from build123d import *

# Parameters (mm, degrees)
EXTRUDE_1_DEPTH          = 85
SKETCH_2_W               = 59.36627173602581
SKETCH_2_H               = 8.418969471425655
EXTRUDE_2_DEPTH          = 25
FILLET_1_R               = 6
FILLET_2_R               = 5
CUT_EXTRUDE_1_REACH      = 117.911
SKETCH_4_R               = 1.499999999999997
SKETCH_7_W               = 35.37461908353682
SKETCH_7_H               = 31.585915090625495
CUT_EXTRUDE_2_DEPTH      = 123.13645897424483
FILLET_3_R               = 5
FILLET_4_R               = 0.5
CUT_EXTRUDE_3_DEPTH      = 192.29117767705227
CUT_EXTRUDE_3_DEPTH_BACK = 192.29117767705227
SKETCH_9_R               = 1.8999999999999981
CUT_EXTRUDE_4_DEPTH      = 27.999999999999996


with BuildPart() as part:
    # 草图1 → 凸台-拉伸1 (new, symmetric)
    with BuildSketch(Plane.XY):
        Polygon((-37.5, 10.529999999999998), (-3.5592322501332707, 10.529999999999998), (-8.298471778986107, 19.8329163418583), (-23.723742156818243, 50.11203580857437), (-19.449282757937613, 61.53100528), (-37.5, 61.53100528), align=None)
    extrude(amount=EXTRUDE_1_DEPTH, both=True)

    # 草图2 → 凸台-拉伸2 (add)
    with BuildSketch(Plane.ZY.offset(37.5)):
        with Locations((0, 54.32152054428719)):
            Rectangle(SKETCH_2_W, SKETCH_2_H)
    extrude(amount=EXTRUDE_2_DEPTH)

    # 圆角1
    fillet_1_edges = [part.edges().sort_by_distance(p)[0] for p in [
        (-37.5, 54.32152054428719, -29.683135868012904),
        (-37.5, 54.32152054428719, 29.683135868012904),
    ]]
    fillet(fillet_1_edges, radius=FILLET_1_R)

    # 圆角2
    fillet_2_edges = [part.edges().sort_by_distance(p)[0] for p in [
        (-62.5, 54.32152054428719, -29.683135868012904),
        (-62.5, 54.32152054428719, 29.683135868012904),
    ]]
    fillet(fillet_2_edges, radius=FILLET_2_R)

    # 草图4 → 切除-拉伸1 (cut, up to next)
    with BuildSketch(Plane(origin=(0, 58.53100528000001, 0), x_dir=(1, 0, 0), z_dir=(0, 1, 0)), mode=Mode.PRIVATE) as cut_extrude_1_sk1:
        with Locations(Location((-47.387450092880144, 14.526154223892442, 0), (0, 0, 270))):
            Circle(SKETCH_4_R)
    cut_extrude_1_tool1 = extrude(cut_extrude_1_sk1.sketch, amount=-CUT_EXTRUDE_1_REACH, mode=Mode.PRIVATE) & part.part
    # 草图4 → 切除-拉伸1 (cut, up to next)
    with BuildSketch(Plane(origin=(0, 58.53100528000001, 0), x_dir=(1, 0, 0), z_dir=(0, 1, 0)), mode=Mode.PRIVATE) as cut_extrude_1_sk2:
        with Locations(Location((-52.407927387117596, 7.976309366063233, 0), (0, 0, 270))):
            Circle(SKETCH_4_R)
    cut_extrude_1_tool2 = extrude(cut_extrude_1_sk2.sketch, amount=-CUT_EXTRUDE_1_REACH, mode=Mode.PRIVATE) & part.part
    # 草图4 → 切除-拉伸1 (cut, up to next)
    with BuildSketch(Plane(origin=(0, 58.53100528000001, 0), x_dir=(1, 0, 0), z_dir=(0, 1, 0)), mode=Mode.PRIVATE) as cut_extrude_1_sk3:
        with Locations(Location((-59.01827910600927, -2.429e-14, 0), (0, 0, 270))):
            Circle(SKETCH_4_R)
    cut_extrude_1_tool3 = extrude(cut_extrude_1_sk3.sketch, amount=-CUT_EXTRUDE_1_REACH, mode=Mode.PRIVATE) & part.part
    # 草图4 → 切除-拉伸1 (cut, up to next)
    with BuildSketch(Plane(origin=(0, 58.53100528000001, 0), x_dir=(1, 0, 0), z_dir=(0, 1, 0)), mode=Mode.PRIVATE) as cut_extrude_1_sk4:
        with Locations(Location((-47.387450092880144, -2.456e-14, 0), (0, 0, 270))):
            Circle(SKETCH_4_R)
    cut_extrude_1_tool4 = extrude(cut_extrude_1_sk4.sketch, amount=-CUT_EXTRUDE_1_REACH, mode=Mode.PRIVATE) & part.part
    # 草图4 → 切除-拉伸1 (cut, up to next)
    with BuildSketch(Plane(origin=(0, 58.53100528000001, 0), x_dir=(1, 0, 0), z_dir=(0, 1, 0)), mode=Mode.PRIVATE) as cut_extrude_1_sk5:
        with Locations(Location((-52.407927387117596, -7.976309366063282, 0), (0, 0, 270))):
            Circle(SKETCH_4_R)
    cut_extrude_1_tool5 = extrude(cut_extrude_1_sk5.sketch, amount=-CUT_EXTRUDE_1_REACH, mode=Mode.PRIVATE) & part.part
    # 草图4 → 切除-拉伸1 (cut, up to next)
    with BuildSketch(Plane(origin=(0, 58.53100528000001, 0), x_dir=(1, 0, 0), z_dir=(0, 1, 0)), mode=Mode.PRIVATE) as cut_extrude_1_sk6:
        with Locations(Location((-47.387450092880144, -14.52615422389249, 0), (0, 0, 270))):
            Circle(SKETCH_4_R)
    cut_extrude_1_tool6 = extrude(cut_extrude_1_sk6.sketch, amount=-CUT_EXTRUDE_1_REACH, mode=Mode.PRIVATE) & part.part
    add(cut_extrude_1_tool1.solids().sort_by_distance((-47.38745, 58.531005, -14.526154))[0], mode=Mode.SUBTRACT)
    add(cut_extrude_1_tool2.solids().sort_by_distance((-52.407927, 58.531005, -7.976309))[0], mode=Mode.SUBTRACT)
    add(cut_extrude_1_tool3.solids().sort_by_distance((-59.018279, 58.531005, 0))[0], mode=Mode.SUBTRACT)
    add(cut_extrude_1_tool4.solids().sort_by_distance((-47.38745, 58.531005, 0))[0], mode=Mode.SUBTRACT)
    add(cut_extrude_1_tool5.solids().sort_by_distance((-52.407927, 58.531005, 7.976309))[0], mode=Mode.SUBTRACT)
    add(cut_extrude_1_tool6.solids().sort_by_distance((-47.38745, 58.531005, 14.526154))[0], mode=Mode.SUBTRACT)

    # 草图7 → 切除-拉伸2 (cut, through all)
    with BuildSketch(Plane(origin=(0, 0, 0), x_dir=(0, 0, -1), z_dir=(1, 0, 0))):
        Polygon((31.999178331290963, 50.11203580857436), (-31.999178331290963, 50.11203580857436), (-31.999178331290956, 18.526120717948867), (31.999178331290956, 18.526120717948867), align=None)
        with Locations((55.6272635970121, 34.319078263261616)):
            Rectangle(SKETCH_7_W, SKETCH_7_H)
        with Locations((-55.6272635970121, 34.319078263261616)):
            Rectangle(SKETCH_7_W, SKETCH_7_H)
    extrude(amount=-CUT_EXTRUDE_2_DEPTH, mode=Mode.SUBTRACT)

    # 圆角3
    fillet_3_edges = [part.edges().sort_by_distance(p)[0] for p in [
        (-22.56637158923609, 18.526120717948867, -37.939954055243696),
        (-30.611871078409123, 50.11203580857436, -73.31457313878052),
        (-22.56637158923609, 18.526120717948867, -73.31457313878052),
        (-30.611871078409123, 50.11203580857437, -37.939954055243696),
        (-30.611871078409123, 50.11203580857437, 37.939954055243696),
        (-22.56637158923609, 18.526120717948867, 37.939954055243696),
        (-22.56637158923609, 18.526120717948867, 73.31457313878052),
        (-30.611871078409123, 50.11203580857436, 73.31457313878052),
        (-22.56637158923609, 18.526120717948867, -31.999178331290956),
        (-30.611871078409123, 50.11203580857436, -31.999178331290963),
        (-22.56637158923609, 18.526120717948867, 31.999178331290956),
        (-30.611871078409123, 50.11203580857436, 31.999178331290963),
    ]]
    fillet(fillet_3_edges, radius=FILLET_3_R)

    # 圆角4
    fillet_4_edges = [part.edges().sort_by_distance(p)[0] for p in [
        (-39.257359312880716, 58.53100528000001, 31.44049518089362),
        (-39.257359312880716, 58.53100528000001, -31.44049518089362),
        (-62.5, 58.53100528000001, 0),
        (-50.5, 58.53100528000001, -29.683135868012904),
        (-50.5, 58.53100528000001, 29.683135868012904),
        (-61.03553390593274, 58.53100528000001, -28.218669773945642),
        (-61.03553390593274, 58.53100528000001, 28.218669773945642),
    ]]
    fillet(fillet_4_edges, radius=FILLET_4_R)

    # 草图8 → 切除-拉伸3 (cut, two sides: drawn at the far end of the back side and taken through both)
    with BuildSketch(Plane.XY.offset(85).offset(-CUT_EXTRUDE_3_DEPTH_BACK)):
        with BuildLine():
            Line((-32.222504901358434, 22.456484131426393), (-21.015514746320488, 22.456484131426393))
            ThreePointArc((-21.015514746320488, 22.456484131426393), (-20.15092452706273, 22.954006517234653), (-20.146640285068184, 23.951516625898744))
            Line((-20.146640285068184, 23.951516625898744), (-31.353630440106134, 43.6218769395131))
            ThreePointArc((-31.353630440106134, 43.6218769395131), (-32.47855717995374, 44.09350738041489), (-33.222504901358434, 43.12684444504075))
            Line((-33.222504901358434, 43.12684444504075), (-33.222504901358434, 23.456484131426393))
            ThreePointArc((-33.222504901358434, 23.456484131426393), (-32.92961168254498, 22.749377350239847), (-32.222504901358434, 22.456484131426393))
        make_face()
    extrude(amount=CUT_EXTRUDE_3_DEPTH + CUT_EXTRUDE_3_DEPTH_BACK, mode=Mode.SUBTRACT)

    # 草图9 → 切除-拉伸4 (cut)
    with BuildSketch(Plane(origin=(0, 18.526120717948867, 0), x_dir=(1, 0, 0), z_dir=(0, 1, 0))):
        with Locations(Location((-32.52765590256421, -19, 0), (0, 0, 270))):
            Circle(SKETCH_9_R)
        with Locations(Location((-32.52765590256421, 19, 0), (0, 0, 270))):
            Circle(SKETCH_9_R)
        with Locations(Location((-17.527655902564213, 19, 0), (0, 0, 270))):
            Circle(SKETCH_9_R)
        with Locations(Location((-17.527655902564213, -19, 0), (0, 0, 270))):
            Circle(SKETCH_9_R)
    extrude(amount=-CUT_EXTRUDE_4_DEPTH, mode=Mode.SUBTRACT)


solid = part.part
Can you work these out from the model? Positions are in its coordinate system, mm. A direction names the side the tool comes from. Give positions to 0.01 mm unless a question says otherwise; leave off trailing zeros. Loops run counter-clockwise (first coordinate to the right, second up) from the corner with the lowest first, then second, coordinate; pieces in that order, holes last. Notation, with made-up numbers: (-26, 44) - (-3, 44) arc R19 cw to (-3, 66) - close; hole circle Ø2 at (56, 89). An arc over 180 degrees is marked (long way). Answer as a JSON object with one key per item and string values.
Q1. Imagine slicing it at A-A on z = 4.5. Write out the boundary of the cut face in (x, y), plus the area to 3 significant figures.
Geometry says:
{"outline": "(-62.5, 50.11) - (-23.72, 50.11) - (-19.45, 61.53) - (-37.5, 61.53) - (-37.5, 58.53) - (-62, 58.53) arc R0.5 ccw to (-62.5, 58.03) - close; (-37.5, 10.53) - (-3.56, 10.53) - (-7.63, 18.53) - (-37.5, 18.53) - close", "area": "647 mm²"}
Q2. Which directions (+Z, -Z, +X, -X, +Y, -Y) give clear straight access to the entire face, cutting with the end or side of a thin tool? Please do faces 1 (the cylindrical face through (-16.244, 14.584, 17.6)), 2 (the flat face through (-6.78, 16.85, 1.19)), 3 (the cylindrical face through (-22.78, 19.95, 71.81)), 4 (the flat face through (-33.223, 33, 35)), 5 (the flat face through (-50, 54, -29.683)).
Geometry says:
{"face 1": "+Y, -Y", "face 2": "+Z, -Z, +X", "face 3": "+X, -X", "face 4": "+Z, -Z", "face 5": "-Z, -X, +Y, -Y"}
Q3. Imagine slicing it at B-B on z = -19. Write out the boundary of the cut face in (x, y).
Geometry says:
{"outline": "(-62.5, 50.11) - (-23.72, 50.11) - (-19.45, 61.53) - (-37.5, 61.53) - (-37.5, 58.53) - (-62, 58.53) arc R0.5 ccw to (-62.5, 58.03) - close; (-37.5, 10.53) - (-34.43, 10.53) - (-34.43, 18.53) - (-37.5, 18.53) - close; (-30.63, 10.53) - (-19.43, 10.53) - (-19.43, 18.53) - (-30.63, 18.53) - close; (-15.63, 10.53) - (-3.56, 10.53) - (-7.63, 18.53) - (-15.63, 18.53) - close"}
Q4. If we mould it in two halves opening along Y, with no side actions, what happens to faces 6 (the cylindrical face through (-16.244, 14.584, -20.4)), 7 (the flat face through (-22, 18.526, 56))? For each: pulls with the +Y half, pulls with the -Y half, needs draft (parallel to the pull), parting line crosses it, or undercut.
Geometry says:
{"face 6": "needs draft", "face 7": "undercut"}
Q5. If I drill on L1, parallel to Z at x = -15, y = 30; L2, parallel to X at y = 15, z = 19; L3, parallel to Y at x = -35, z = -8.5, over which ranges is the centre line in solid material (lowest first)?
Geometry says:
{"L1": "-85 to -73.31, -37.94 to -32, 32 to 37.94, 73.31 to 85", "L2": "-37.5 to -34.43, -30.63 to -19.43, -15.63 to -5.84", "L3": "10.53 to 18.53, 50.11 to 61.53"}
Q6. Will these pins go through, and if not, where does the flat tip stop? P1, Ø6.5, axis at x = -48, y = 55.5, coming from the -Z side; P2, Ø1.5, axis at x = -56, y = 56, coming from the +Z side; P3, Ø3.5, axis at x = -52.41, z = 7.98, coming from the -Y side.
Geometry says:
{"P1": "z = -29.68", "P2": "z = 29.68", "P3": "y = 50.11"}
Q7. Imagine slicing it at C-C on y = 29. Give the number of separate pieces and of enclosed holes in the cut face, plus the area to 3 significant figures.
Geometry says:
{"separate pieces": "8", "enclosed holes": "0", "area": "505 mm²"}
